Can you work these out from the model? Positions are in its coordinate system, mm. A direction names the side the tool comes from. Round coordinates to 2 decimals unless told otherwise and drop trailing zeros. Loops run counter-clockwise (first coordinate to the right, second up) from the corner with the lowest first, then second, coordinate; pieces in that order, holes last.
```python
from build123d import *

# Parameters (mm, degrees)
SKETCH1_W           = 2.54
SKETCH1_H           = 2.54
BOSS_EXTRUDE1_DEPTH = 2.54
BOSS_EXTRUDE2_DEPTH = 1.397
BOSS_EXTRUDE2_TAPER = 15
FILLET1_R           = 0.381
FILLET2_R           = 0.127
SKETCH3_R           = 1.27
CUT_EXTRUDE1_DEPTH  = 0.381
CUT_EXTRUDE1_TAPER  = 30


with BuildPart() as part:
    # Sketch1 → Boss-Extrude1 (new body)
    with BuildSketch(Plane(origin=(0, 0, 0), x_dir=(1, 0, 0), z_dir=(0, 1, 0))):
        Rectangle(SKETCH1_W, SKETCH1_H)
    extrude(amount=BOSS_EXTRUDE1_DEPTH)

    # Sketch2 → Boss-Extrude2 (add)
    with BuildSketch(Plane(origin=(0, 2.54, 0), x_dir=(1, 0, 0), z_dir=(0, 1, 0))):
        with BuildLine():
            Line((6.345965274, 1.102171866), (0.946447911, 4.1932578))
            ThreePointArc((0.946447911, 4.1932578), (0, 4.445), (-0.946447911, 4.1932578))
            Line((-0.946447911, 4.1932578), (-6.345965274, 1.102171866))
            ThreePointArc((-6.345965274, 1.102171866), (-6.985, 0), (-6.345965274, -1.102171866))
            Line((-6.345965274, -1.102171866), (-0.946447911, -4.1932578))
            ThreePointArc((-0.946447911, -4.1932578), (0, -4.445), (0.946447911, -4.1932578))
            Line((0.946447911, -4.1932578), (6.345965274, -1.102171866))
            ThreePointArc((6.345965274, -1.102171866), (6.985, 0), (6.345965274, 1.102171866))
        make_face()
    extrude(amount=BOSS_EXTRUDE2_DEPTH, taper=BOSS_EXTRUDE2_TAPER)

    # Fillet1
    fillet1_edges = [part.edges().sort_by_distance(p)[0] for p in [
        (0, 3.937, -4.070674978),
        (-3.460233293, 3.937, -2.322856165),
        (-6.610674978, 3.937, 0),
        (-3.460233293, 3.937, 2.322856165),
        (0, 3.937, 4.070674978),
        (3.460233293, 3.937, 2.322856165),
        (6.610674978, 3.937, 0),
        (3.460233293, 3.937, -2.322856165),
    ]]
    fillet(fillet1_edges, radius=FILLET1_R)

    # Fillet2
    fillet2_edges = [part.edges().sort_by_distance(p)[0] for p in [
        (0, 2.54, -4.445),
        (-3.646206592, 2.54, -2.647714833),
        (-6.985, 2.54, 0),
        (-3.646206592, 2.54, 2.647714833),
        (0, 2.54, 4.445),
        (3.646206592, 2.54, 2.647714833),
        (6.985, 2.54, 0),
        (3.646206592, 2.54, -2.647714833),
    ]]
    fillet(fillet2_edges, radius=FILLET2_R)

    # Sketch3 → Cut-Extrude1 (cut)
    with BuildSketch(Plane(origin=(0, 3.937, 0), x_dir=(1, 0, 0), z_dir=(0, 1, 0))):
        Circle(SKETCH3_R)
    extrude(amount=-CUT_EXTRUDE1_DEPTH, taper=CUT_EXTRUDE1_TAPER, mode=Mode.SUBTRACT)


solid = part.part
```
(1) For pin 1 (1 mm diameter, centred on y = 2.5, z = -1.5, fed in from +X); pin 2 (1 mm diameter, centred on x = -4, z = 2.5, fed in from -Y); pin 3 (0.8 mm diameter, centred on x = 0, y = 0.5, fed in from +Z), each with a flat end and sliding along its axis, tell me the tip position at first contact or that it passes through.
(2) Suppose I cut it at A-A (y = 1.25). Write out the boundary of the cut face in (x, z), then the cut area to 3 significant figures.
(3) Which directions (+Z, -Z, +X, -X, +Y, -Y) give clear straight access to the entire face, cutting with the end or side of a thin tool? Please do faces 1 (the flat face through (0, 1, -1.27)), 2 (the flat face through (0, 0, 0)), 3 (the flat face through (0, 1, 1.27)).
(4) If I drill on line 1 (Y direction, x = -2.5, z = -1.5); line 2 (X direction, y = 3.75, z = 0.25); line 3 (X direction, y = 1.85, z = -0.5), over which ranges is the centre line in solid material (lowest first)?
(5) We'd pull the mould along X, two halves only. Please class faces 4 (the flat face through (1.27, 1, 0)), 5 (the flat face through (-1.27, 1, 0)), 6 (the flat face through (0, 3.556, 0)): released by +X, released by -X, zero draft, split by the parting line, or undercut.
Check result:
1. pin 1: stops at x = 6.4
1. pin 2: stops at y = 2.54
1. pin 3: stops at z = 1.27
2. outline: (-1.27, -1.27) - (1.27, -1.27) - (1.27, 1.27) - (-1.27, 1.27) - close
2. area: 6.45 mm2
3. face 1: -Z, +X, -X, -Y
3. face 2: +Z, -Z, +X, -X, -Y
3. face 3: +Z, +X, -X, -Y
4. line 1: y = 2.54 to 3.94
4. line 2: x = -6.61 to -1.13, 1.13 to 6.61
4. line 3: x = -1.27 to 1.27
5. face 4: released by +X
5. face 5: released by -X
5. face 6: undercut
